```python
from build123d import *

# Parameters (mm, degrees)
F1_DEPTH = 63.5
F2_DEPTH = 25.4
F3_DEPTH = 7.9375
F5_R     = 6.35


with BuildPart() as f1:
    # F0 (on Front) → F1 (new body, symmetric)
    with BuildSketch(Plane.XZ):
        Polygon((22.2249999642, 9.525), (-41.275, 9.525), (-41.275, -9.525), (41.275, -9.525), (41.275, 9.525), align=None)
    extrude(amount=F1_DEPTH, both=True)

    # F0 (on Front) → F2 (join, symmetric)
    with BuildSketch(Plane.XZ):
        with BuildLine():
            Line((22.2249999642, 27.1821387616), (22.2249999642, 9.525))
            Line((22.2249999642, 9.525), (41.275, 9.525))
            Line((41.275, 9.525), (41.275, 27.1821387616))
            ThreePointArc((41.275, 27.1821387616), (46.8066352935, 39.2249968754), (59.5465504312, 42.8752))
            Line((59.5465504312, 42.8752), (60.325, 42.8752))
            Line((60.325, 42.8752), (60.325, 61.8121879463))
            add(Edge.make_bspline(
                [(53.5827816682, 61.924484406), (55.9043140785, 61.9405018001), (58.157358995, 61.9025346921), (60.325, 61.8121879463)],
                knots=[107.4684002997, 107.4684002997, 107.4684002997, 107.4684002997, 113.9637235604, 113.9637235604, 113.9637235604, 113.9637235604], degree=3))
            ThreePointArc((53.5827816682, 61.924484406), (31.2237514489, 50.5826785752), (22.2249999642, 27.1821387616))
        make_face()
        with BuildLine():
            add(Edge.make_bspline(
                [(60.325, 61.8121879463), (61.0334566794, 61.7826596455), (61.7327905274, 61.7475361607), (62.422410954, 61.7068735214)],
                knots=[113.9637235604, 113.9637235604, 113.9637235604, 113.9637235604, 116.0866097479, 116.0866097479, 116.0866097479, 116.0866097479], degree=3))
            Line((60.325, 61.8121879463), (60.325, 42.8752))
            Line((60.325, 42.8752), (81.01685845, 42.8752))
            Line((81.01685845, 42.8752), (81.01685845, 61.9251988828))
            Line((81.01685845, 61.9251988828), (60.7102529284, 61.9251988828))
            ThreePointArc((60.7102529284, 61.9251988828), (61.5676808741, 61.8266148465), (62.422410954, 61.7068735214))
        make_face()
    extrude(amount=F2_DEPTH, both=True)

    # F0 (on Front) → F3 (join, symmetric)
    with BuildSketch(Plane.XZ):
        with BuildLine():
            add(Edge.make_bspline(
                [(-41.275, 9.525), (-41.9877743947, 46.6159944116), (15.1718567055, 61.659468539), (53.5827816682, 61.924484406)],
                knots=[0, 0, 0, 0, 107.4684002997, 107.4684002997, 107.4684002997, 107.4684002997], degree=3))
            Line((-41.275, 9.525), (22.2249999642, 9.525))
            Line((22.2249999642, 9.525), (22.2249999642, 27.1821387616))
            ThreePointArc((22.2249999642, 27.1821387616), (31.2237514489, 50.5826785752), (53.5827816682, 61.924484406))
        make_face()
    extrude(amount=F3_DEPTH, both=True)

    # F0 (on Front) → F4 (revolve)
    with BuildSketch(Plane.XZ):
        Polygon((111.125, 63.3849346732), (81.01685845, 63.3849346732), (81.01685845, 61.9251988828), (81.01685845, 42.8752), (81.01685845, 34.8099346732), (111.125, 34.8099346732), align=None)
    revolve(axis=Axis((81.01685845, 0, 49.0974346732), (0, 0, 1)))

    # F5
    f5_edges = [f1.edges().sort_by_distance(p)[0] for p in [
        (-41.275, -63.5, 0),
        (41.275, -63.5, 0),
        (41.275, 63.5, 0),
        (-41.275, 63.5, 0),
    ]]
    fillet(f5_edges, radius=F5_R)


solid = f1.part
```
CAD build for the part. Positions are in the model's coordinates, mm. A direction names the side the tool comes from. Round coordinates to 2 decimals unless told otherwise and drop trailing zeros. Loops run counter-clockwise (first coordinate to the right, second up) from the corner with the lowest first, then second, coordinate; pieces in that order, holes last. Notation, with made-up numbers: (-33.5, 30.5) - (-10.5, 30.5) arc R15 cw to (-10.5, 35.5) - close; hole circle Ø9 at (20.25, 10.5). An arc over 180 degrees is marked (long way). Return JSON: item names as keys, results as strings. Group by question number.
Q1. Band-saw the part on A-A on z = -4. Give the cut face in (x, y) (3 decimals).
Q2. Tool access for faces 1 (the face through (62, -25, 61.925)), 2 (the face through (39, 25.4, 36)), 3 (the face through (-41.275, -1, 0)), 4 (the face through (81, 0, 34.81)), 5 (the face through (61, 24, 42.875)): list every direction of +Z, -Z, +X, -X, +Y, -Y with a clear straight run to the whole face (end or side of a thin tool).
Q3. Drill centre lines: line 1 along Y through (x, z) = (35.5, 5.5); line 2 along Y through (x, z) = (-10, 46); line 3 along Z through (x, y) = (81, -30). Where is each one in solid material? Low to high. Write a range as [from, to].
Q4. Band-saw the part on B-B on y = 42. Give the cut face in (x, z) (3 decimals).
Q5. Flat gauge pins, fed straight in: pin 1 Ø6 at (x, z) = (26.5, 54.5) entering from +Y; pin 2 Ø4.5 at (x, y) = (63.5, 22.5) entering from -Z; pin 3 Ø6 at (y, z) = (-21.5, 34.5) entering from -X. Where does each tip first touch, or does it go through?
Q6. Band-saw the part on C-C on x = 80.5. Give the cut face in (y, z), plus the area to 3 significant figures.
Solutions:
{
 "1": {"outline": "(-41.275, -57.15) arc R6.35 ccw to (-34.925, -63.5) - (34.925, -63.5) arc R6.35 ccw to (41.275, -57.15) - (41.275, 57.15) arc R6.35 ccw to (34.925, 63.5) - (-34.925, 63.5) arc R6.35 ccw to (-41.275, 57.15) - close"},
 "2": {"face 1": "+Z, -X, -Y", "face 2": "+Z, -X, +Y", "face 3": "+Z, -Z, -X, +Y, -Y", "face 4": "-Z, +X, +Y, -Y", "face 5": "-Z, +Y"},
 "3": {"line 1": "y = [-63.47, 63.47]", "line 2": "y = [-7.94, 7.94]", "line 3": "z = [34.81, 63.38]"},
 "4": {"outline": "(-41.275, -9.525) - (41.275, -9.525) - (41.275, 9.525) - (-41.275, 9.525) - close"},
 "5": {"pin 1": "stops at y = 7.94", "pin 2": "stops at z = 34.81", "pin 3": "stops at x = 22.49"},
 "6": {"outline": "(-30.1, 34.81) - (30.1, 34.81) - (30.1, 63.38) - (-30.1, 63.38) - close", "area": "1,720 mm^2"}
}
